from build123d import *

# Parameters (mm, degrees)
SKETCH1_R           = 5
BOSS_EXTRUDE1_DEPTH = 7
SKETCH2_R           = 2.75
CUT_EXTRUDE1_DEPTH  = 35.759746835


with BuildPart() as part:
    # Sketch1 → Boss-Extrude1 (new, symmetric)
    with BuildSketch(Plane.XY):
        Polygon((-21, 0), (21, 0), (21, 6), (9, 6), (9, 32.8), (-9, 32.8), (-9, 6), (-21, 6), align=None)
        with Locations((0, 20)):
            Circle(SKETCH1_R, mode=Mode.SUBTRACT)
    extrude(amount=BOSS_EXTRUDE1_DEPTH, both=True)

    # Sketch2 → Cut-Extrude1 (cut, through all)
    with BuildSketch(Plane(origin=(0, 6, 0), x_dir=(1, 0, 0), z_dir=(0, 1, 0))):
        with Locations(Location((-16, 0, 0), (0, 0, 180))):
            Circle(SKETCH2_R)
        with Locations(Location((16, 0, 0), (0, 0, 180))):
            Circle(SKETCH2_R)
    extrude(amount=-CUT_EXTRUDE1_DEPTH, mode=Mode.SUBTRACT)


solid = part.part
The listing builds one solid part. Answer for the finished solid, in the listing's coordinates (mm). A direction names the side the tool comes from. Give positions to 0.01 mm unless a question says otherwise; leave off trailing zeros. Write each loop counter-clockwise with the first axis right and the second up, starting at its lowest first coordinate (ties: lowest second). Pieces come first, ordered by that corner, then holes.
1) For a pull along Z with two mould halves and no side action, classify faces 4 (the face through (18.747, 3.042, 0.121)), 5 (the face through (-13.6, 6, 1.7)), 6 (the face through (0, 13, -7)) as pulls with the +Z half, pulls with the -Z half, needs draft (parallel to the pull), parting line crosses it, or undercut.
2) Section B-B (x = -16) is taken. Write down the section's boundary in (y, z), and give its area (3 significant figures).
3) Given P1, Ø6, axis at x = -18, z = -1.5, coming from the +Y side; P2, Ø1, axis at y = 26, z = 4.5, coming from the -X side, each flat-ended and moving along its own axis, determine where each tip first touches the part or whether it passes through.
4) Section C-C (z = 0) is taken. Write down the section's boundary in (x, y), and give its area (3 significant figures).
5) Section D-D (z = 4.5) is taken. Write down the section's boundary in (x, y), and give its area (3 significant figures).
6) Find the intervals of material crossed by L1, parallel to X at y = 4, z = -0.5; L2, parallel to Y at x = 0, z = -1.75; L3, parallel to Z at x = 16, y = 4, in increasing order.
7) Section A-A (y = 20) is taken. Write down the section's boundary in (x, z).
8) A tool of negligible diameter and unlimited length cuts with its end or side. For faces 1 (the face through (12, 6, 0)), 2 (the face through (21, 3, 0)), 3 (the face through (-9, 20, 0)), from which of +Z, -Z, +X, -X, +Y, -Y can it reach the whole face along a straight path? Write none if from no direction.
Response:
1. face 4: undercut
1. face 5: needs draft
1. face 6: pulls with the -Z half
2. outline: (0, -7) - (6, -7) - (6, -2.75) - (0, -2.75) - close; (0, 2.75) - (6, 2.75) - (6, 7) - (0, 7) - close
2. area: 51.0 mm2
3. P1: stops at y = 6
3. P2: stops at x = -9
4. outline: (-21, 0) - (-18.75, 0) - (-18.75, 6) - (-21, 6) - close; (-13.25, 0) - (13.25, 0) - (13.25, 6) - (9, 6) - (9, 32.8) - (-9, 32.8) - (-9, 6) - (-13.25, 6) - close; (18.75, 0) - (21, 0) - (21, 6) - (18.75, 6) - close; hole circle Ø10 at (0, 20)
4. area: 590 mm2
5. outline: (-21, 0) - (21, 0) - (21, 6) - (9, 6) - (9, 32.8) - (-9, 32.8) - (-9, 6) - (-21, 6) - close; hole circle Ø10 at (0, 20)
5. area: 656 mm2
6. L1: x = -21 to -18.7, -13.3 to 13.3, 18.7 to 21
6. L2: y = 0 to 15, 25 to 32.8
6. L3: z = -7 to -2.75, 2.75 to 7
7. outline: (-9, -7) - (-5, -7) - (-5, 7) - (-9, 7) - close; (5, -7) - (9, -7) - (9, 7) - (5, 7) - close
8. face 1: +Z, -Z, +X, +Y
8. face 2: +Z, -Z, +X, +Y, -Y
8. face 3: +Z, -Z, -X, +Y
